Input: part model. Units: mm. Frame: model coordinates. A direction names the side the tool comes from. Give positions to 0.01 mm unless a question says otherwise; leave off trailing zeros. Loops run counter-clockwise (first coordinate to the right, second up) from the corner with the lowest first, then second, coordinate; pieces in that order, holes last. Notation, with made-up numbers: M -15.75,87 L 1.25,87 A29 ccw 1.25,109 Z; hole C 58,53 d9. An arc over 180 degrees is marked long. Use CSV: the item, a comma, the result in double quotes. Start each with the question number.
from build123d import *

# Parameters (mm, degrees)
F0_W      = 76.2
F0_H      = 25.4
F0_W_2    = 69.85
F0_H_2    = 19.05
F1_DEPTH  = 5.08
F2_W      = 7.62
F2_H      = 0.635
F3_DEPTH  = 1.778
F4_W      = 0.635
F4_H      = 2.54
F5_DEPTH  = 1.778
F6_W      = 0.1422071991
F6_H      = 0.635
F7_DEPTH  = 0.762
F8_R      = 0.4959508544
F9_DEPTH  = 7.4777928009
F10_W     = 0.0690778879
F10_H     = 0.635
F11_DEPTH = 0.762
F12_R     = 0.4959508544
F13_DEPTH = 7.5509221121
F14_W     = 0.095821996
F14_H     = 0.635
F15_DEPTH = 0.762
F16_R     = 0.4959508544
F17_DEPTH = 7.524178004
F18_W     = 0.0717212304
F18_H     = 0.635
F19_DEPTH = 0.762
F20_R     = 0.4959508544
F21_DEPTH = 7.5482787696
F22_W     = 0.635
F22_H     = 0.1154780363
F23_DEPTH = 0.762
F24_R     = 0.4959508544
F25_DEPTH = 2.4245219637
F26_W     = 0.635
F26_H     = 0.1073694763
F27_DEPTH = 0.762
F28_R     = 0.4959508544
F29_DEPTH = 2.4326305237


with BuildPart() as f1:
    # F0 (on Front) → F1 (new body)
    with BuildSketch(Plane.XZ):
        with Locations((8.76239234, 5.4013291374)):
            Rectangle(F0_W, F0_H)
        with Locations((8.76239234, 5.4013291374)):
            Rectangle(F0_W_2, F0_H_2, mode=Mode.SUBTRACT)
    extrude(amount=F1_DEPTH)

    # F2 (on face) → F3 (join)
    with BuildSketch(Plane.XZ.offset(5.08)):
        with Locations((26.22489234, 17.4663291374)):
            Rectangle(F2_W, F2_H)
        with Locations((26.22489234, 15.5613291374)):
            Rectangle(F2_W, F2_H)
        with Locations((-8.70010766, 17.4663291374)):
            Rectangle(F2_W, F2_H)
        with Locations((-8.70010766, 15.5613291374)):
            Rectangle(F2_W, F2_H)
    extrude(amount=F3_DEPTH)

    # F4 (on face) → F5 (join)
    with BuildSketch(Plane.XZ.offset(5.08)):
        with Locations((9.71489234, -5.7111708626)):
            Rectangle(F4_W, F4_H)
        with Locations((7.80989234, -5.7111708626)):
            Rectangle(F4_W, F4_H)
    extrude(amount=F5_DEPTH)

    # F6 (on face) → F7 (join)
    with BuildSketch(Plane.XZ.offset(6.858)):
        with Locations((-12.4390040605, 17.4663291374)):
            Rectangle(F6_W, F6_H)
    extrude(amount=F7_DEPTH)

    # F8 (on face) → F9 (join, through all)
    with BuildSketch(Plane.YZ.offset(-12.367900461)):
        with Locations((-7.239, 17.4663291374)):
            Circle(F8_R)
    extrude(amount=F9_DEPTH)

    # F10 (on face) → F11 (join)
    with BuildSketch(Plane.XZ.offset(6.858)):
        with Locations((-12.4755687161, 15.5613291374)):
            Rectangle(F10_W, F10_H)
    extrude(amount=F11_DEPTH)

    # F12 (on face) → F13 (join, through all)
    with BuildSketch(Plane.YZ.offset(-12.4410297722)):
        with Locations((-7.239, 15.5613291374)):
            Circle(F12_R)
    extrude(amount=F13_DEPTH)

    # F14 (on face) → F15 (join)
    with BuildSketch(Plane.XZ.offset(6.858)):
        with Locations((29.986981342, 17.4663291374)):
            Rectangle(F14_W, F14_H)
    extrude(amount=F15_DEPTH)

    # F16 (on face) → F17 (join, through all)
    with BuildSketch(Plane(origin=(29.939070344, 0, 0), x_dir=(0, -1, 0), z_dir=(-1, 0, 0))):
        with Locations((7.239, 17.4663291374)):
            Circle(F16_R)
    extrude(amount=F17_DEPTH)

    # F18 (on face) → F19 (join)
    with BuildSketch(Plane.XZ.offset(6.858)):
        with Locations((29.9990317248, 15.5613291374)):
            Rectangle(F18_W, F18_H)
    extrude(amount=F19_DEPTH)

    # F20 (on face) → F21 (join, through all)
    with BuildSketch(Plane(origin=(29.9631711096, 0, 0), x_dir=(0, -1, 0), z_dir=(-1, 0, 0))):
        with Locations((7.239, 15.5613291374)):
            Circle(F20_R)
    extrude(amount=F21_DEPTH)

    # F22 (on face) → F23 (join)
    with BuildSketch(Plane.XZ.offset(6.858)):
        with Locations((7.80989234, -4.4989098807)):
            Rectangle(F22_W, F22_H)
    extrude(amount=F23_DEPTH)

    # F24 (on face) → F25 (join, through all)
    with BuildSketch(Plane(origin=(0, 0, -4.5566488989), x_dir=(1, 0, 0), z_dir=(0, 0, -1))):
        with Locations((7.80989234, 7.239)):
            Circle(F24_R)
    extrude(amount=F25_DEPTH)

    # F26 (on face) → F27 (join)
    with BuildSketch(Plane.XZ.offset(6.858)):
        with Locations((9.71489234, -4.4948556007)):
            Rectangle(F26_W, F26_H)
    extrude(amount=F27_DEPTH)

    # F28 (on face) → F29 (join, through all)
    with BuildSketch(Plane(origin=(0, 0, -4.5485403389), x_dir=(1, 0, 0), z_dir=(0, 0, -1))):
        with Locations((9.71489234, 7.239)):
            Circle(F28_R)
    extrude(amount=F29_DEPTH)


solid = f1.part
Item 1: Section D-D (x = 17). Output: boundary loops of the cut face in (y, z), then the cut area to 3 significant figures.
Item 2: Section C-C (y = -2.75). Output: boundary loops of the cut face in (x, z), then the cut area to 3 significant figures.
Item 3: Material intervals for line 1 (X direction, y = -3.5, z = 13.5); line 2 (Z direction, x = -25, y = -4); line 3 (Y direction, x = 20.5, z = -5), sorted ascending.
Item 4: Mould query, pull axis X, two halves, no side actions, for faces 3 (the flat face through (6, 0, -5)), 4 (the flat face through (7.492, -6, -6)), 5 (the flat face through (8, -3, 14.926)). Classes: +X half, -X half, draft (parallel to the pull), parting line (faces both ways), or undercut.
Item 5: Section B-B (z = 10.25). Output: boundary loops of the cut face in (x, y).
Item 6: Section A-A (x = -10.5). Output: boundary loops of the cut face in (y, z), then the cut area to 3 significant figures.
Item 7: Set-up query: faces 1 (the flat face through (-29.338, -3, 5)), 2 (the flat face through (8, -3, -4.124)). Return all of +Z, -Z, +X, -X, +Y, -Y with unobstructed straight access to the full face (end or side cutting, diameter ignored); none if empty.
Item 8: First-contact query: pin 1 Ø2 at (x, y) = (-8.5, -6.5) entering from -Z; pin 2 Ø0.8 at (y, z) = (-6.5, 17.5) entering from +X; pin 3 Ø2 at (y, z) = (-7, 7.5) entering from +X; pin 4 Ø0.8 at (y, z) = (-6, 17) entering from -X. Flat tips, straight axial feed; report the tip coordinate or a pass-through.
Recorded:
1,outline,"M -5.08,-7.3 L 0,-7.3 L 0,-4.12 L -5.08,-4.12 Z; M -5.08,14.93 L 0,14.93 L 0,18.1 L -5.08,18.1 Z"
1,area,"32.3 mm²"
2,outline,"M -29.34,-7.3 L 46.86,-7.3 L 46.86,18.1 L -29.34,18.1 Z; hole M -26.16,-4.12 L 43.69,-4.12 L 43.69,14.93 L -26.16,14.93 Z"
2,area,"605 mm²"
3,line 1,"-29.34 to -26.16, 43.69 to 46.86"
3,line 2,"-7.3 to -4.12, 14.93 to 18.1"
3,line 3,"-5.08 to 0"
4,face 3,"draft"
4,face 4,"-X half"
4,face 5,"undercut"
5,outline,"M -29.34,-5.08 L -26.16,-5.08 L -26.16,0 L -29.34,0 Z; M 43.69,-5.08 L 46.86,-5.08 L 46.86,0 L 43.69,0 Z"
6,outline,"M -6.86,15.24 L -5.08,15.24 L -5.08,14.93 L 0,14.93 L 0,18.1 L -5.08,18.1 L -5.08,17.78 L -6.86,17.78 A0.5 ccw long -6.86,17.15 L -5.08,17.15 L -5.08,15.88 L -6.86,15.88 A0.5 ccw long Z; M -5.08,-7.3 L 0,-7.3 L 0,-4.12 L -5.08,-4.12 Z"
6,area,"36.0 mm²"
7,face 1,"+Z, -Z, -X, +Y, -Y"
7,face 2,"+Y, -Y"
8,pin 1,"z = 15.07"
8,pin 2,"x = 30.03"
8,pin 3,"through"
8,pin 4,"x = -12.51"
